Source: CAD feature listing. Evaluate the final solid. Frame: model axes, mm. A direction names the side the tool comes from. Round coordinates to 2 decimals unless told otherwise and drop trailing zeros. Order: outer loops, then holes, each group sorted by start corner. A loop starts at its lowest first (then second) coordinate and runs counter-clockwise, first axis right, second up. Notation, with made-up numbers: M -15.5,-18.5 L -10.5,-18.5 A9 ccw -10.5,-12.5 Z; hole C -23,55 d6. An arc over 180 degrees is marked long. Answer as CSV lines item,"result". Start each with the question number.
Item 1: Section query A-A on y = 7.75. Return the cut outline in (x, z) (3 decimals).
Item 2: Line query: line 1 (X direction, y = 7, z = 4.75) (3 decimals); line 2 (X direction, y = 2.5, z = 8) (3 decimals); line 3 (Z direction, x = 10.25, y = 4). Output: solid intervals per line, ascending. Write a range as [from, to].
Item 3: First-contact query: P1, Ø5, axis at x = 10, y = 5.5, coming from the -Z side (3 decimals); P2, Ø1.5, axis at y = 3.5, z = 0.5, coming from the -X side; P3, Ø1, axis at x = -2.5, z = 5.5, coming from the -Y side. Flat tips, straight axial feed; report the tip coordinate or a pass-through.
Item 4: Set-up query: faces 4 (the face through (1.997, 4.93, 1.907)), 5 (the face through (11.13, 6.51, -4.9)), 6 (the face through (-7.82, 3.76, -4.39)), 7 (the face through (-2.69, 0.477, 8.755)). Return all of +Z, -Z, +X, -X, +Y, -Y with unobstructed straight access to the full face (end or side cutting, diameter ignored); none if empty.
Item 5: Pull-direction query (Y, two-part tool) for faces 1 (the face through (2.69, 0.477, 8.688)), 2 (the face through (-0.09, 9.55, -12.22)), 3 (the face through (7.82, 6.24, -4.39)); classes: +Y half, -Y half, draft (parallel to the pull), parting line (faces both ways), or undercut.
Autodesk Inventor part; units mm, degrees
ref_plane "Work Plane1" through (0, 5, 0) normal (0, 1, 0) x (1, 0, 0)
ref_plane "Work Plane2" through (0, 1.5875, -6.35) normal (1, 0, 0) x (0, 0, -1)
ref_plane "YZ Plane" through (0, 0, 0) normal (1, 0, 0) x (0, 1, 0)
sketch "Sketch1" plane through (0, 0, 0) normal (0, 1, 0) x (-1, 0, 0)
  circle A0 centre (0, 0) radius 2.65
  line L0 (2.65, -1.53) -> (0, -3.06)
  line L1 (0, -3.06) -> (-2.65, -1.53)
  line L2 (-2.65, -1.53) -> (-2.65, 1.53)
  line L3 (-2.65, 1.53) -> (0, 3.06)
  line L4 (0, 3.06) -> (2.65, 1.53)
  line L5 (2.65, 1.53) -> (2.65, -1.53)
  line L6 (1.325, 12.7) -> (-1.325, 12.7)
  line L7 (-12.7, -3.2069) -> (-12.7, -6.35)
  line L8 (-6.35, -12.7) -> (6.35, -12.7)
  line L9 (12.7, -6.35) -> (12.7, -3.2069)
  line L10 (12.7, 12.7) -> (-12.7, -12.7) construction
  line L11 (-12.7, 12.7) -> (12.7, -12.7) construction
  arc A1 (-12.7, -6.35) -> (-6.35, -12.7) centre (-6.35, -6.35) ccw
  arc A2 (6.35, -12.7) -> (12.7, -6.35) centre (6.35, -6.35) ccw
  line L12 (1.325, 2.295) -> (1.325, 12.7)
  line L13 (-1.325, 2.295) -> (-1.325, 12.7)
  circle A3 centre (0, 0) radius 4.445
  line L14 (6.3181, 3.1431) -> (6.35, 3.1431)
  line L15 (-6.3181, 3.1431) -> (-6.35, 3.1431)
  arc A4 (-6.35, 3.1431) -> (-12.7, -3.2069) centre (-6.35, -3.2069) ccw
  arc A5 (12.7, -3.2069) -> (6.35, 3.1431) centre (6.35, -3.2069) ccw
  line L16 (-3.1431, 6.3181) -> (-3.1431, 11.1252)
  line L17 (-1.5683, 12.7) -> (-1.325, 12.7)
  line L18 (1.325, 12.7) -> (1.5683, 12.7)
  line L19 (3.1431, 11.1252) -> (3.1431, 6.3181)
  arc A6 (-6.3181, 3.1431) -> (-3.1431, 6.3181) centre (-6.3181, 6.3181) ccw
  arc A7 (3.1431, 6.3181) -> (6.3181, 3.1431) centre (6.3181, 6.3181) ccw
  arc A8 (3.1431, 11.1252) -> (1.5683, 12.7) centre (1.5683, 11.1252) ccw
  arc A9 (-1.5683, 12.7) -> (-3.1431, 11.1252) centre (-1.5683, 11.1252) ccw
  point P0 (2.65, 0)
  point P1 (3.1431, 3.1431)
  point P2 (-3.1431, 3.1431)
  point P3 (-12.7, 3.1431)
  point P4 (3.1431, 12.7)
  dimension "d0" = 5.3
  dimension "d1" = 25.4
  dimension "d2" = 25.4
  dimension "d4" = 8.89
  dimension "d5" = 6.35
  dimension "d6" = 3.175
  dimension "d7" = 1.5748
extrude "Extrusion1" add sketch "Sketch1" along normal blind 10 contours L5 L4 L12 A3 L13 L3 L2 L1 L0 | L12 L18 A8 L19 A7 L14 A5 L9 A2 L8 A1 L7 A4 L15 A6 L16 A9 L17 L13 A3
fillet "Fillet1" radius 1.5875 34 edges at (-10.8401, 10, 1.2832) (-6.334, 10, 3.1431) (-4.073, 10, 4.073) (-3.1431, 10, 8.7216) (-2.6818, 10, 12.2388) (-1.4466, 10, 12.7) (-10.8401, 10, -10.8401) (0, 10, -12.7) (10.8401, 10, -10.8401) (12.7, 10, -4.7785) (10.8401, 10, 1.2832) (6.334, 10, 3.1431) (4.073, 10, 4.073) (3.1431, 10, 8.7216) (2.6818, 10, 12.2388) (1.4466, 10, 12.7) (-12.7, 10, -4.7785) (-10.8401, 0, 1.2832) (-6.334, 0, 3.1431) (-4.073, 0, 4.073) (-3.1431, 0, 8.7216) (-2.6818, 0, 12.2388) (-1.4466, 0, 12.7) (-10.8401, 0, -10.8401) (0, 0, -12.7) (10.8401, 0, -10.8401) (12.7, 0, -4.7785) (10.8401, 0, 1.2832) (6.334, 0, 3.1431) (4.073, 0, 4.073) (3.1431, 0, 8.7216) (2.6818, 0, 12.2388) (1.4466, 0, 12.7) (-12.7, 0, -4.7785)
sketch "Sketch2" plane through (-3.1431, 1.5875, 11.1252) normal (-1, 0, 0) x (0, 0, 1)
  line L0 (-4.8071, 0) -> (-4.8071, 6.825) construction
  line L1 (-4.8071, 3.4125) -> (0, 3.4125) construction
  line L2 (0, 0) -> (0, 6.825) construction
  line L3 (-4.8071, 0) -> (0, 0) construction
  line L4 (-2.4036, 0) -> (-2.4036, 6.825) construction
  line L5 (-4.8071, 6.825) -> (0, 6.825) construction
  circle A0 centre (-2.4036, 3.4125) radius 1.15
  circle A1 centre (-2.4036, 3.4125) radius 1.75
  point P0 (-11.1252, -1.5875)
  dimension "d11" = 2.3
  dimension "d12" = 3.5
extrude "Extrusion2" cut sketch "Sketch2" against normal up to surface (1.8181 mm away) contours A0 | A1
extrude "Extrusion3" cut sketch "Sketch2" against normal up to surface (6.2862 mm away) contours A0
ref_plane "Work Plane1" through (0, 5, 0) normal (0, 1, 0) x (1, 0, 0)
sketch "Sketch3" plane through (0, 5, 0) normal (0, 1, 0) x (1, 0, 0)
  line L0 (-12.7508, 4.6668) -> (-6.1607, 4.6668)
  line L1 (-5.0471, 5.128) -> (-2.6519, 7.5232)
  line L2 (0, 13.8984) -> (0, -13.9494) construction
  line L3 (12.7508, 4.6668) -> (6.1607, 4.6668)
  line L4 (5.0471, 5.128) -> (2.6519, 7.5232)
  arc A0 (5.0471, 5.128) -> (6.1607, 4.6668) centre (6.1607, 6.2416) ccw
  arc A1 (-6.1607, 4.6668) -> (-5.0471, 5.128) centre (-6.1607, 6.2416) ccw
  point P0 (0, 0)
  point P1 (-5.5084, 4.6668)
  point P2 (5.5084, 4.6668)
  dimension "d17" = 135
  dimension "d18" = 1.5748
sketch "Sketch4" plane through (12.7, 1.5875, -6.35) normal (1, 0, 0) x (0, 0, -1)
  circle A0 centre (-1.6832, 3.4125) radius 1.27
  line L0 (7.5484, 3.4125) -> (-20.2994, 3.4125) construction
  point P0 (-6.35, -1.5875)
  dimension "d19" = 2.54
sweep "Sweep1" cut profiles "Sketch4" path "Sketch3" path curves L3 A0 L4
ref_plane "Work Plane2" through (0, 1.5875, -6.35) normal (1, 0, 0) x (0, 0, -1)
chamfer "Chamfer1" distance 0.508 distance2 3.175 1 edges at (12.7, 5, -3.3968) measured on face at (12.7, 2.3048, -4.7923)
mirror "Mirror1" about plane through (0, 1.5875, -6.35) normal (1, 0, 0) of "Sweep1"
chamfer "Chamfer2" distance 0.508 distance2 3.175 1 edges at (-12.7, 5, -3.3968) measured on face at (-12.7, 7.6952, -4.7923)
properties part number "Bad Intake Bracket v2"
Results:
1,outline,"M -12.7,-6.35 A6.35 ccw -6.35,-12.7 L 6.35,-12.7 A6.35 ccw 12.7,-6.35 L 12.7,-3.207 A6.35 ccw 6.35,3.143 L 6.318,3.143 A3.175 cw 3.143,6.318 L 3.143,11.125 A1.575 ccw 1.568,12.7 L 1.325,12.7 L 1.325,2.295 L 2.65,1.53 L 2.65,-1.53 L 0,-3.06 L -2.65,-1.53 L -2.65,1.53 L -1.325,2.295 L -1.325,12.7 L -1.568,12.7 A1.575 ccw -3.143,11.125 L -3.143,6.318 A3.175 cw -6.318,3.143 L -6.35,3.143 A6.35 ccw -12.7,-3.207 Z"
2,line 1,"[-3.557, -1.325], [1.325, 3.557]"
2,line 2,"[-3.143, -1.325], [1.325, 3.143]"
2,line 3,"[-11.36, -5.63], [-3.71, 1.8]"
3,P1,"z = -12.595"
3,P2,"x = -11.97"
3,P3,"y = 0.04"
4,face 4,"+Y, -Y"
4,face 5,"+X"
4,face 6,"-X"
4,face 7,"+Z, -X, -Y"
5,face 1,"-Y half"
5,face 2,"+Y half"
5,face 3,"undercut"
